Can you work these out from the model? Positions are in its coordinate system, mm. A direction names the side the tool comes from. Coordinates: 2 decimals unless noted, no trailing zeros. Order: outer loops, then holes, each group sorted by start corner. A loop starts at its lowest first (then second) coordinate and runs counter-clockwise, first axis right, second up. Notation, with made-up numbers: (70, 74) -> (98, 74) arc R17 cw to (98, 96) -> close; hole circle Ø8 at (86, -14.75). An arc over 180 degrees is marked (long way). Answer in a Markdown table with one row per item.
```python
from build123d import *

# Parameters (mm, degrees)
SKETCH1_W           = 31.8
SKETCH1_H           = 15.9
BOSS_EXTRUDE1_DEPTH = 3
SKETCH2_R           = 2.475
BOSS_EXTRUDE2_DEPTH = 1.9
SKETCH3_W           = 28.8
SKETCH3_H           = 12.9
CUT_EXTRUDE1_DEPTH  = 2


with BuildPart() as part:
    # Sketch1 → Boss-Extrude1 (new body)
    with BuildSketch(Plane(origin=(0, 0, 0), x_dir=(1, 0, 0), z_dir=(0, 1, 0))):
        with Locations((15.9, -7.95)):
            Rectangle(SKETCH1_W, SKETCH1_H)
    extrude(amount=BOSS_EXTRUDE1_DEPTH)

    # Sketch2 → Boss-Extrude2 (add)
    with BuildSketch(Plane(origin=(0, 3, 0), x_dir=(1, 0, 0), z_dir=(0, 1, 0))):
        with Locations(Location((3.975, -3.975, 0), (0, 0, 90))):
            Circle(SKETCH2_R)
        with Locations(Location((11.925, -3.975, 0), (0, 0, 90))):
            Circle(SKETCH2_R)
        with Locations(Location((19.875, -3.975, 0), (0, 0, 90))):
            Circle(SKETCH2_R)
        with Locations(Location((27.825, -3.975, 0), (0, 0, 90))):
            Circle(SKETCH2_R)
        with Locations(Location((27.825, -11.925, 0), (0, 0, 90))):
            Circle(SKETCH2_R)
        with Locations(Location((19.875, -11.925, 0), (0, 0, 90))):
            Circle(SKETCH2_R)
        with Locations(Location((11.925, -11.925, 0), (0, 0, 90))):
            Circle(SKETCH2_R)
        with Locations(Location((3.975, -11.925, 0), (0, 0, 90))):
            Circle(SKETCH2_R)
    extrude(amount=BOSS_EXTRUDE2_DEPTH)

    # Sketch3 → Cut-Extrude1 (cut)
    with BuildSketch(Plane.XZ):
        with Locations((15.9, 7.95)):
            Rectangle(SKETCH3_W, SKETCH3_H)
    extrude(amount=-CUT_EXTRUDE1_DEPTH, mode=Mode.SUBTRACT)


solid = part.part
```
(1) We'd pull the mould along X, two halves only. Please class faces 1 (the flat face through (20, 4.9, 12)), 2 (the cylindrical face through (4.923, 3.937, 9.639)): +X half, -X half, draft (parallel to the pull), parting line (faces both ways), or undercut.
Response values:
| item | result |
|---|---|
| face 1 | draft |
| face 2 | undercut |
(2) On a 3-axis mill with a long thin cutter (end or side, diameter ignored), from which of +Z, -Z, +X, -X, +Y, -Y can I reach the whole of each face in a straight line? I mean faces 3 (the cylindrical face through (30.02, 3.94, 10.78)), 4 (the flat face through (17, 0, 1)), 5 (the flat face through (16, 1, 14.4)). Say none if no direction works.
Response values:
| item | result |
|---|---|
| face 3 | +Y |
| face 4 | +Z, -Z, +X, -X, -Y |
| face 5 | -Y |
(3) Suppose I cut it at A-A (y = 0.9). Please give me the cut outline in (x, z), and give its area (3 significant figures).
Response values:
| item | result |
|---|---|
| outline | (0, 0) -> (31.8, 0) -> (31.8, 15.9) -> (0, 15.9) -> close; hole (1.5, 1.5) -> (30.3, 1.5) -> (30.3, 14.4) -> (1.5, 14.4) -> close |
| area | 134 mm2 |
(4) Suppose I cut it at C-C (x = 23). Please give me the cut outline in (y, z).
Response values:
| item | result |
|---|---|
| outline | (0, 0) -> (3, 0) -> (3, 15.9) -> (0, 15.9) -> (0, 14.4) -> (2, 14.4) -> (2, 1.5) -> (0, 1.5) -> close |
(5) I need wall thicknesses on line 1 (X direction, y = 0.3, z = 9.75); line 2 (Z direction, x = 14, y = 1.25); line 3 (X direction, y = 4.2, z = 2.75). Which ranges of each line are inside material? Lowest first, please. Write a range as [from, to].
Response values:
| item | result |
|---|---|
| line 1 | [0, 1.5], [30.3, 31.8] |
| line 2 | [0, 1.5], [14.4, 15.9] |
| line 3 | [1.82, 6.13], [9.77, 14.08], [17.72, 22.03], [25.67, 29.98] |
(6) Suppose I cut it at B-B (y = 3.5). Please give me the cut outline in (x, z) (3 decimals), and give its area (3 significant figures).
Response values:
| item | result |
|---|---|
| outline | circle Ø4.95 at (3.975, 3.975); circle Ø4.95 at (3.975, 11.925); circle Ø4.95 at (11.925, 3.975); circle Ø4.95 at (11.925, 11.925); circle Ø4.95 at (19.875, 3.975); circle Ø4.95 at (19.875, 11.925); circle Ø4.95 at (27.825, 3.975); circle Ø4.95 at (27.825, 11.925) |
| area | 154 mm2 |
(7) Suppose I cut it at D-D (z = 3.5). Please give me the cut outline in (x, y).
Response values:
| item | result |
|---|---|
| outline | (0, 0) -> (1.5, 0) -> (1.5, 2) -> (30.3, 2) -> (30.3, 0) -> (31.8, 0) -> (31.8, 3) -> (30.25, 3) -> (30.25, 4.9) -> (25.4, 4.9) -> (25.4, 3) -> (22.3, 3) -> (22.3, 4.9) -> (17.45, 4.9) -> (17.45, 3) -> (14.35, 3) -> (14.35, 4.9) -> (9.5, 4.9) -> (9.5, 3) -> (6.4, 3) -> (6.4, 4.9) -> (1.55, 4.9) -> (1.55, 3) -> (0, 3) -> close |
(8) Will this pin go through, and if not, where does the flat tip stop? pin 1 Ø1 at (x, z) = (13.5, 3.5) entering from -Y.
Response values:
| item | result |
|---|---|
| pin 1 | y = 2 |
